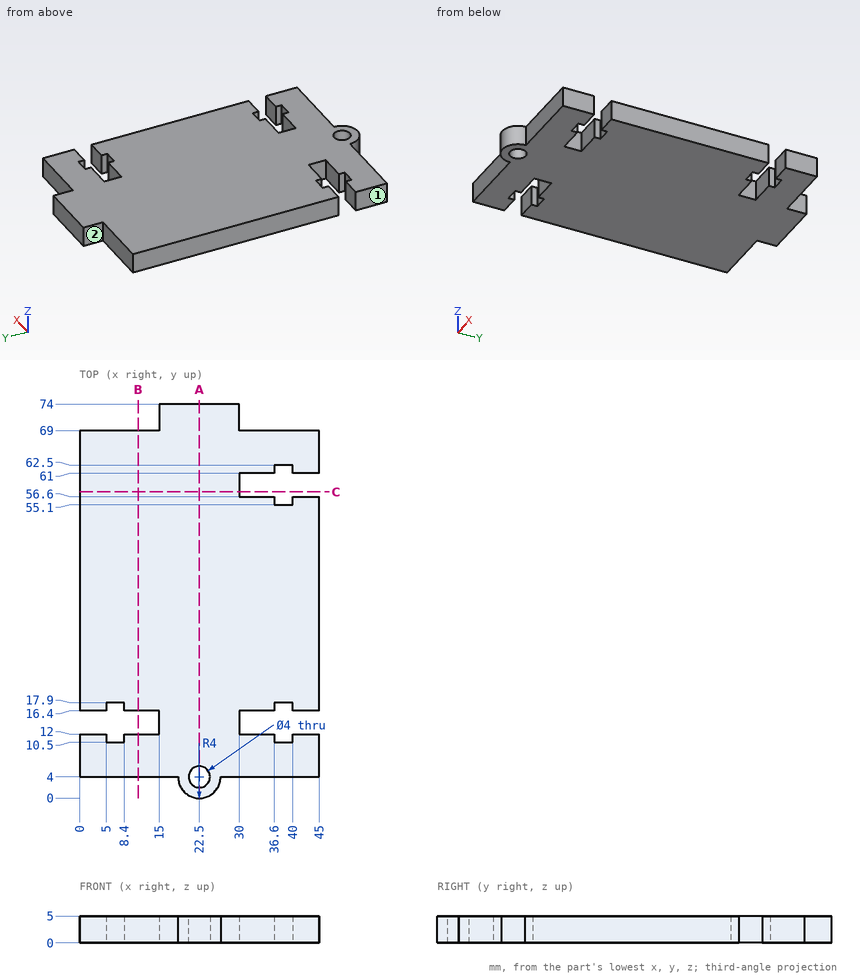
Can you work these out from the drawing? Everything is in mm from the part's minimum corner. A direction names the side the tool comes from. Give positions to 0.01 mm unless a question says otherwise; leave off trailing zeros. Order: outer loops, then holes, each group sorted by start corner. A loop starts at its lowest first (then second) coordinate and runs counter-clockwise, first axis right, second up. Notation, with made-up numbers: M 67.5,-16.5 L 82.5,-16.5 A21 ccw 82.5,-2.5 Z; hole C 87,-23.5 d10. An arc over 180 degrees is marked long. One line per item, written item: value.
Item 1: For the marked faces 1 and 2, which set-ups out of +Z, -Z, +X, -X, +Y, -Y let a thin tool reach every point of the face, with its end or its side?
Verdict:
face 1: +Z, -Z, -X, +Y, -Y
face 2: +Z, -Z, -X, +Y
Item 2: For pin 1 (2.5 mm diameter, centred on x = 41.5, z = 3.5, fed in from +Y); pin 2 (1 mm diameter, centred on x = 7, z = 1.5, fed in from -Y), each with a flat end and sliding along its axis, tell me the tip position at first contact or that it passes through.
Verdict:
pin 1: y = 69
pin 2: y = 4
Item 3: If we section it at A-A on x = 22.5: Write out the boundary of the cut face in (y, z).
Verdict:
outline: M 0,0 L 2,0 L 2,5 L 0,5 Z; M 6,0 L 74,0 L 74,5 L 6,5 Z
Item 4: Please list where these lines run through material, in increasing order: line 1 (Y direction, x = 31, z = 0.55); line 2 (Y direction, x = 39.5, z = 0.95); line 3 (Y direction, x = 22.5, z = 2.95).
Verdict:
line 1: 4 to 12, 16.4 to 56.6, 61 to 69
line 2: 4 to 10.5, 17.9 to 55.1, 62.5 to 69
line 3: 0 to 2, 6 to 74
Item 5: If we section it at C-C on y = 57.5: Write out the boundary of the cut face in (x, z), and give its area (3 significant figures).
Verdict:
outline: M 0,0 L 30,0 L 30,5 L 0,5 Z
area: 150 mm2
Item 6: If we section it at B-B on x = 11: Write out the boundary of the cut face in (y, z).
Verdict:
outline: M 4,0 L 12,0 L 12,5 L 4,5 Z; M 16.4,0 L 69,0 L 69,5 L 16.4,5 Z
